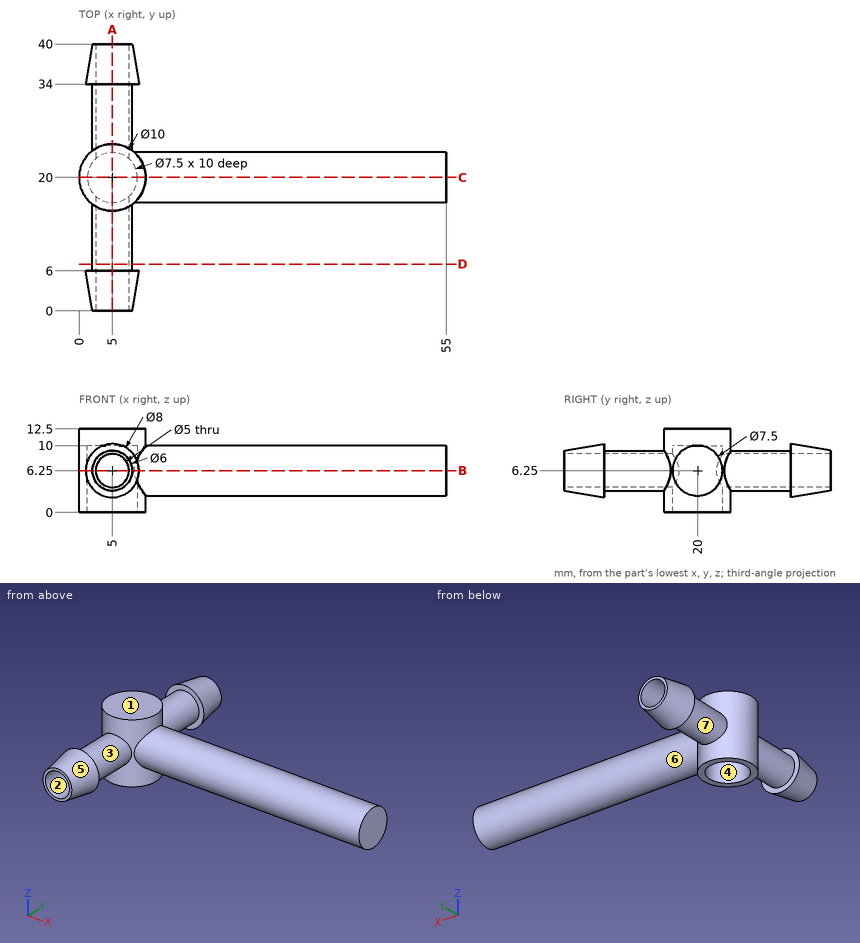
Source: three-view drawing plus pictorial views. Frame: mm from the lowest corner of the part. A direction names the side the tool comes from. Give positions to 0.01 mm unless a question says otherwise; leave off trailing zeros. Loops run counter-clockwise (first coordinate to the right, second up) from the corner with the lowest first, then second, coordinate; pieces in that order, holes last. Notation, with made-up numbers: (33.5, -14) -> (80.5, -14) arc R16 ccw to (80.5, 6) -> close; hole circle Ø6 at (81.25, 22). An arc over 180 degrees is marked (long way). Put each result on its own line as item: value. Start each with the question number.
1) Cut plane D-D (y = 7). Return loops of the section in (x, z).
2) Material intervals for probe 1 along Z at (x, y) = (5, 13); probe 2 along X at (y, z) = (38, 4.5); probe 3 along Z at (x, y) = (5, 4), sorted ascending.
3) Draft query along Z for the marked faces 1, 2 and 3. Return one class per face: released by +Z, released by -Z, zero draft, split by the parting line, or undercut.
4) Cut plane C-C (y = 20). Return loops of the section in (x, z), then the cut area to 4 significant figures.
5) Cut plane A-A (x = 5). State how many separate pieces and enclosed holes the cut face has, then the cut area to 3 significant figures.
6) Cut plane B-B (z = 6.25). Return loops of the section in (x, y).
7) Reachability of the marked faces 4, 5, 6 and 7 from +Z, -Z, +X, -X, +Y, -Y: full face, straight path, thin tool, end or side. Return the list, or none.
8) Contact query for flat-ended pins moving along their axis: P1, Ø4.5, axis at x = 5, y = 20, coming from the -Z side; P2, Ø2, axis at x = 30.5, z = 7.5, coming from the -Y side; P3, Ø1, axis at x = 11, y = 35, coming from the -Z side; P4, Ø12, axis at x = 41, y = 14.5, coming from the +Z side. Output: stop coordinate, or through.
Results are:
1. outline: circle Ø6 at (5, 6.25); hole circle Ø5 at (5, 6.25)
2. probe 1: z = 3.25 to 3.75, 8.75 to 9.25
2. probe 2: x = 2.16 to 3.21, 6.79 to 7.84
2. probe 3: z = 2.58 to 3.75, 8.75 to 9.92
3. face 1: released by +Z
3. face 2: undercut
3. face 3: split by the parting line
4. outline: (0, 0) -> (1.25, 0) -> (1.25, 10) -> (8.75, 10) -> (8.75, 0) -> (10, 0) -> (10, 2.5) -> (55, 2.5) -> (55, 10) -> (10, 10) -> (10, 12.5) -> (0, 12.5) -> close
4. area: 387.5 mm2
5. separate pieces: 3
5. enclosed holes: 0
5. area: 79.5 mm2
6. outline: (1, 6) -> (2, 0) -> (2.5, 0) -> (2.5, 17.2) arc R3.75 cw to (2.5, 22.8) -> (2.5, 40) -> (2, 40) -> (1, 34) -> (2, 34) -> (2, 24) arc R5 ccw to (2, 16) -> (2, 6) -> close; (7.5, 0) -> (8, 0) -> (9, 6) -> (8, 6) -> (8, 16) arc R5 ccw to (8.31, 16.25) -> (55, 16.25) -> (55, 23.75) -> (8.31, 23.75) arc R5 ccw to (8, 24) -> (8, 34) -> (9, 34) -> (8, 40) -> (7.5, 40) -> (7.5, 22.8) arc R3.75 cw to (7.5, 17.2) -> close
7. face 4: -Z
7. face 5: -Y
7. face 6: +X
7. face 7: none
8. P1: stops at z = 10
8. P2: stops at y = 16.26
8. P3: passes through
8. P4: stops at z = 10
